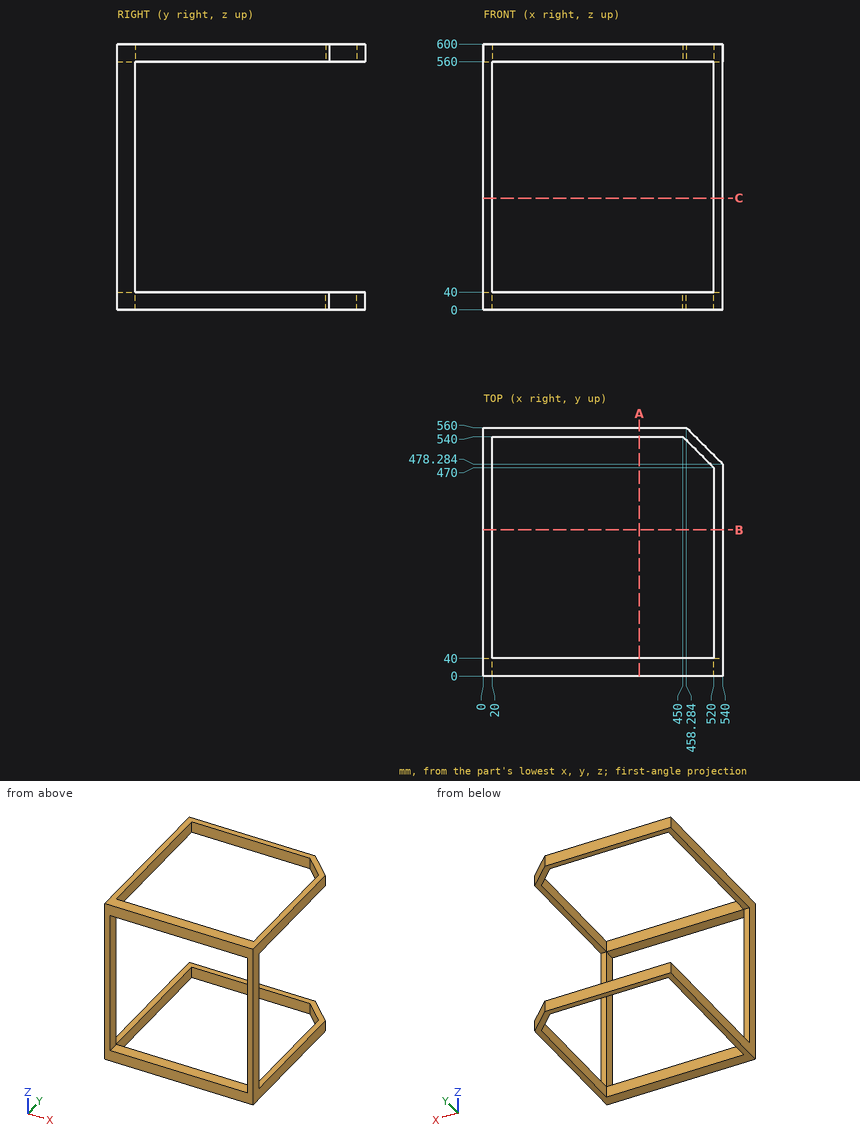
Check sheet for the drawn part. Datum: minimum x, y, z corner. Units: mm. Round coordinates to 2 decimals unless told otherwise and drop trailing zeros. Loops run counter-clockwise (first coordinate to the right, second up) from the corner with the lowest first, then second, coordinate; pieces in that order, holes last. Notation, with made-up numbers: (49.25, -8.5) - (94.25, -8.5) arc R19 cw to (94.25, 14.5) - close; hole circle Ø6 at (17.25, 59.5). An arc over 180 degrees is marked (long way). Answer as a JSON object with one key per item and string values. Group by question number.
Q1. Gauge pin test, flat end, axial feed: P1, Ø6, axis at x = 526.5, z = 409.5, coming from the +Y side. Record the tip position at first contact, or that the pin passes through.
Q2. Sectioned sample at A-A, the plane x = 352. Enter the section's corners in (y, z), plus the area to 3 significant figures.
Q3. Sectioned sample at B-B, the plane y = 329.5. Enter the section's corners in (x, z).
Q4. Sectioned sample at C-C, the plane z = 252. Enter the section's corners in (x, y), plus the area to 3 significant figures.
Q5. Scan lines: line 1 along X through (y, z) = (400.5, 32); line 2 along Z through (x, y) = (130.5, 30). Record each from-to range of solid material in increasing order. Write a range as [from, to].
Solution:
{
 "1": {"P1": "stops at y = 40"},
 "2": {"outline": "(0, 0) - (40, 0) - (40, 40) - (0, 40) - close; (0, 560) - (40, 560) - (40, 600) - (0, 600) - close; (540, 0) - (560, 0) - (560, 40) - (540, 40) - close; (540, 560) - (560, 560) - (560, 600) - (540, 600) - close", "area": "4,800 mm²"},
 "3": {"outline": "(0, 0) - (20, 0) - (20, 40) - (0, 40) - close; (0, 560) - (20, 560) - (20, 600) - (0, 600) - close; (520, 0) - (540, 0) - (540, 40) - (520, 40) - close; (520, 560) - (540, 560) - (540, 600) - (520, 600) - close"},
 "4": {"outline": "(0, 0) - (20, 0) - (20, 40) - (0, 40) - close; (520, 0) - (540, 0) - (540, 40) - (520, 40) - close", "area": "1,600 mm²"},
 "5": {"line 1": "x = [0, 20], [520, 540]", "line 2": "z = [0, 40], [560, 600]"}
}
